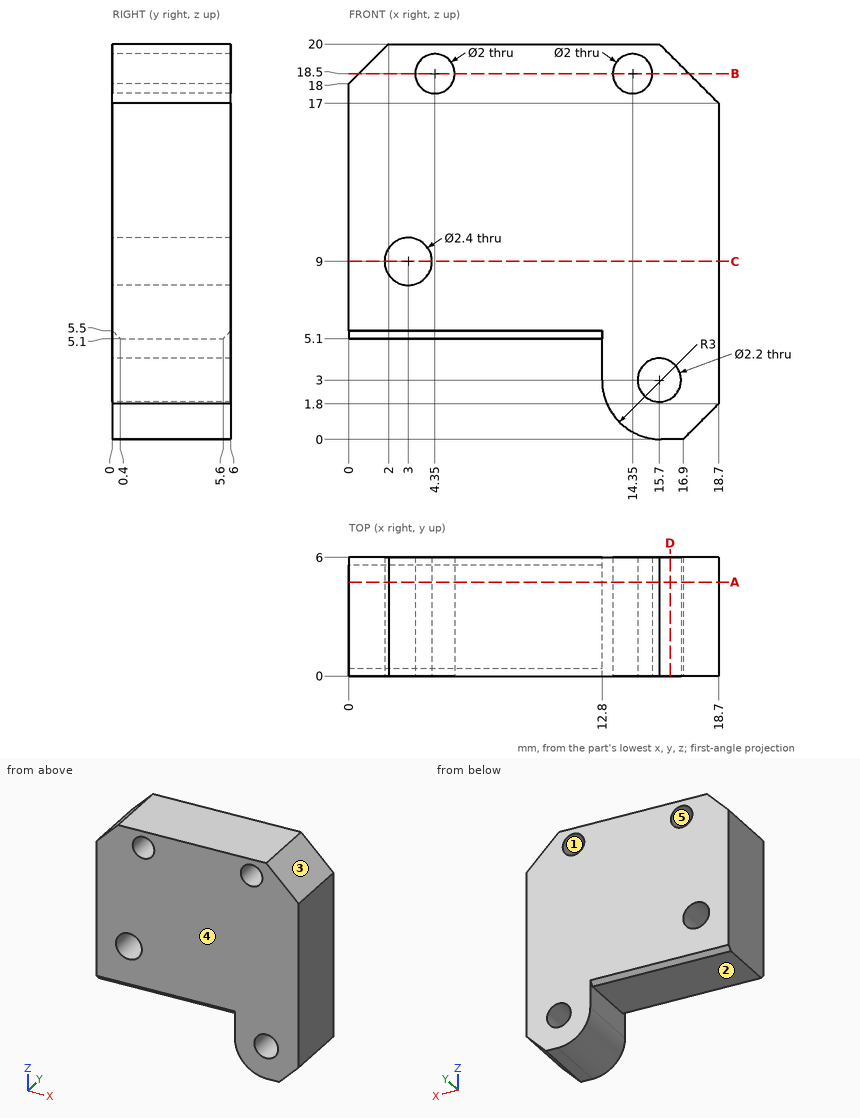
Geometry check sheet. Reference: drawing and pictorial views, mm from the part's lowest x, y, z. A direction names the side the tool comes from. Coordinates: 2 decimals unless noted, no trailing zeros. Write each loop counter-clockwise with the first axis right and the second up, starting at its lowest first coordinate (ties: lowest second). Pieces come first, ordered by that corner, then holes. Notation, with made-up numbers: M 43,52.5 L 100,52.5 A18 cw 100,86.5 Z; hole C 67,30.25 d11. An arc over 180 degrees is marked long. One line per question, with ' | ' between items.
1) Sectioned sample at A-A on y = 4.75. Record the cut outline in (x, z).
Solutions:
outline: M 0,5.1 L 12.8,5.1 L 12.8,3 A3 ccw 15.8,0 L 16.9,0 L 18.7,1.8 L 18.7,17 L 15.7,20 L 2,20 L 0,18 Z; hole C 3,9 d2.4; hole C 4.35,18.5 d2; hole C 14.35,18.5 d2; hole C 15.7,3 d2.2
2) Sectioned sample at B-B on z = 18.5. Record the cut outline in (x, y), then the cut area to 3 significant figures.
Solutions:
outline: M 0.5,0 L 3.35,0 L 3.35,6 L 0.5,6 Z; M 5.35,0 L 13.35,0 L 13.35,6 L 5.35,6 Z; M 15.35,0 L 17.2,0 L 17.2,6 L 15.35,6 Z | area: 76.2 mm^2
3) Access from +Z, -Z, +X, -X, +Y, -Y to the whole of each face (thin tool, end or side, straight path). Record for the marked faces 1 and 2.
Solutions:
face 1: +Y, -Y | face 2: -Z, -X, +Y, -Y
4) Release check for a two-part mould opening along Z. For the marked faces 3, 4 and 5 record: +Z half, -Z half, draft (parallel to the pull), parting line (faces both ways), or undercut.
Solutions:
face 3: +Z half | face 4: draft | face 5: undercut
5) Depth check by flat-ended pin: pin 1 Ø2 at (y, z) = (1, 4) entering from -X; pin 2 Ø3 at (x, z) = (3, 9) entering from -Y; pin 3 Ø1.2 at (x, z) = (4.35, 18.5) entering from +Y; pin 4 Ø1 at (x, y) = (13.5, 1) entering from -Z. Enter the tip coordinate at first touch or a pass-through.
Solutions:
pin 1: x = 12.8 | pin 2: y = 0 | pin 3: through | pin 4: z = 0.6
6) Material ranges on L1, parallel to X at y = 2.25, z = 3; L2, parallel to X at y = 5, z = 9; L3, parallel to Z at x = 3, y = 2.75, recorded low to high.
Solutions:
L1: 12.8 to 14.6, 16.8 to 18.7 | L2: 0 to 1.8, 4.2 to 18.7 | L3: 5.1 to 7.8, 10.2 to 20
7) Sectioned sample at D-D on x = 16.25. Record the cut outline in (y, z).
Solutions:
outline: M 0,0 L 6,0 L 6,2.05 L 0,2.05 Z; M 0,3.95 L 6,3.95 L 6,19.45 L 0,19.45 Z
8) Sectioned sample at C-C on z = 9. Record the cut outline in (x, y).
Solutions:
outline: M 0,0 L 1.8,0 L 1.8,6 L 0,6 Z; M 4.2,0 L 18.7,0 L 18.7,6 L 4.2,6 Z
